```python
from build123d import *

# Parameters (mm, degrees)
SKETCH_1_R          = 25
EXTRUDE_1_DEPTH     = 30
SKETCH_2_R          = 20
CUT_EXTRUDE_1_DEPTH = 30
SKETCH_3_R          = 20
CUT_EXTRUDE_2_DEPTH = 40
SKETCH_4_R          = 15
CUT_EXTRUDE_4_DEPTH = 200


with BuildPart() as part:
    # 草图1 → 凸台-拉伸1 (new, symmetric)
    with BuildSketch(Plane(origin=(0, 0, 0), x_dir=(0, 0, -1), z_dir=(1, 0, 0))):
        Circle(SKETCH_1_R)
    extrude(amount=EXTRUDE_1_DEPTH, both=True)

    # 草图2 → 切除-拉伸1 (cut, symmetric)
    with BuildSketch(Plane(origin=(0, 0, 0), x_dir=(0, 0, -1), z_dir=(1, 0, 0))):
        Circle(SKETCH_2_R)
    extrude(amount=CUT_EXTRUDE_1_DEPTH, both=True, mode=Mode.SUBTRACT)

    # 草图3 → 切除-拉伸2 (cut)
    with BuildSketch(Plane(origin=(0, 0, 0), x_dir=(1, 0, 0), z_dir=(0, 1, 0))):
        with Locations(Location((0, 0, 0), (0, 0, 90))):
            Circle(SKETCH_3_R)
    extrude(amount=CUT_EXTRUDE_2_DEPTH, mode=Mode.SUBTRACT)

    # 草图4 → 切除-拉伸4 (cut)
    with BuildSketch(Plane(origin=(0, 0, 0), x_dir=(1, 0, 0), z_dir=(0, 1, 0))):
        with Locations(Location((0, 0, 0), (0, 0, 270))):
            Circle(SKETCH_4_R)
    extrude(amount=-CUT_EXTRUDE_4_DEPTH, mode=Mode.SUBTRACT)


solid = part.part
```
Input: part model. Units: mm. Frame: model coordinates. Give positions to 0.01 mm unless a question says otherwise; leave off trailing zeros. Order: outer loops, then holes, each group sorted by start corner. A loop starts at its lowest first (then second) coordinate and runs counter-clockwise, first axis right, second up. Notation, with made-up numbers: M -32,9 L -3,9 A31 ccw -3,35 Z; hole C -26,50.5 d10. An arc over 180 degrees is marked long. Return JSON: item names as keys, results as strings.
Item 1: Cut plane B-B (x = 0). Return loops of the section in (y, z).
Solutions:
{"outline": "M -20,-15 A25 ccw 15,-20 L 0,-20 A20 cw -13.23,-15 Z; M -20,15 L -13.23,15 A20 cw 0,20 L 15,20 A25 ccw Z"}
Item 2: Cut plane D-D (z = 19). Return loops of the section in (x, y) (3 decimals), then the cut area to 3 significant figures.
Solutions:
{"outline": "M -30,-16.248 L 30,-16.248 L 30,-6.245 L -30,-6.245 Z; M -30,6.245 L -6.245,6.245 L -6.245,16.248 L -30,16.248 Z; M 6.245,6.245 L 30,6.245 L 30,16.248 L 6.245,16.248 Z", "area": "1,080 mm^2"}
Item 3: Cut plane C-C (y = 3.5). Return loops of the section in (x, z), then the cut area to 3 significant figures.
Solutions:
{"outline": "M -30,-24.75 L 30,-24.75 L 30,-19.69 L 3.5,-19.69 A20 cw -3.5,-19.69 L -30,-19.69 Z; M -30,19.69 L -3.5,19.69 A20 cw 3.5,19.69 L 30,19.69 L 30,24.75 L -30,24.75 Z", "area": "605 mm^2"}
Item 4: Cut plane A-A (z = 0). Return loops of the section in (x, y), then the cut area to 3 significant figures.
Solutions:
{"outline": "M -30,-25 L -15,-25 L -15,-20 L -30,-20 Z; M -30,20 L -20,20 L -20,25 L -30,25 Z; M 15,-25 L 30,-25 L 30,-20 L 15,-20 Z; M 20,20 L 30,20 L 30,25 L 20,25 Z", "area": "250 mm^2"}
Item 5: Ray query, probe 1 along Y at (x, z) = (3, -15); probe 2 along Y at (x, z) = (-21.5, 11); probe 3 along Z at (x, y) = (-25, -15.5). Return the intervals inside material, ascending.
Solutions:
{"probe 1": "-20 to -13.23", "probe 2": "-22.45 to -16.7, 16.7 to 22.45", "probe 3": "-19.62 to -12.64, 12.64 to 19.62"}
Item 6: Pull-direction query (Z, two-part tool) for faces 1 (the cylindrical face through (0, -15, 20)), 2 (the cylindrical face through (-13.31, -19.03, 6.92)), 3 (the cylindrical face through (8.713, 14.294, 18.002)), 4 (the flat face through (30, 17, 11)); classes: +Z half, -Z half, draft (parallel to the pull), parting line (faces both ways), or undercut.
Solutions:
{"face 1": "parting line", "face 2": "undercut", "face 3": "undercut", "face 4": "draft"}
Item 7: First-contact query: P1, Ø24, axis at x = 0, z = 0, coming from the -Y side; P2, Ø10, axis at x = -0.5, y = 9, coming from the +Z side; P3, Ø6, axis at x = -8, y = 1, coming from the +Z side; P4, Ø4, axis at x = 12, y = 9.5, coming from the +Z side. Flat tips, straight axial feed; report the tip coordinate or a pass-through.
Solutions:
{"P1": "through", "P2": "z = 24.68", "P3": "z = 25", "P4": "z = 23.85"}
